For this review, use the dimensioned drawing (mm, ordinates from the lowest corner) and the shaded views. Coordinates: 2 decimals unless noted, no trailing zeros. Write each loop counter-clockwise with the first axis right and the second up, starting at its lowest first coordinate (ties: lowest second). Pieces come first, ordered by that corner, then holes. Notation, with made-up numbers: M 45,55.5 L 94,55.5 A33 cw 94,88.5 Z; hole C -25.5,-17.75 d10. An arc over 180 degrees is marked long. One line per question, with ' | ' between items.
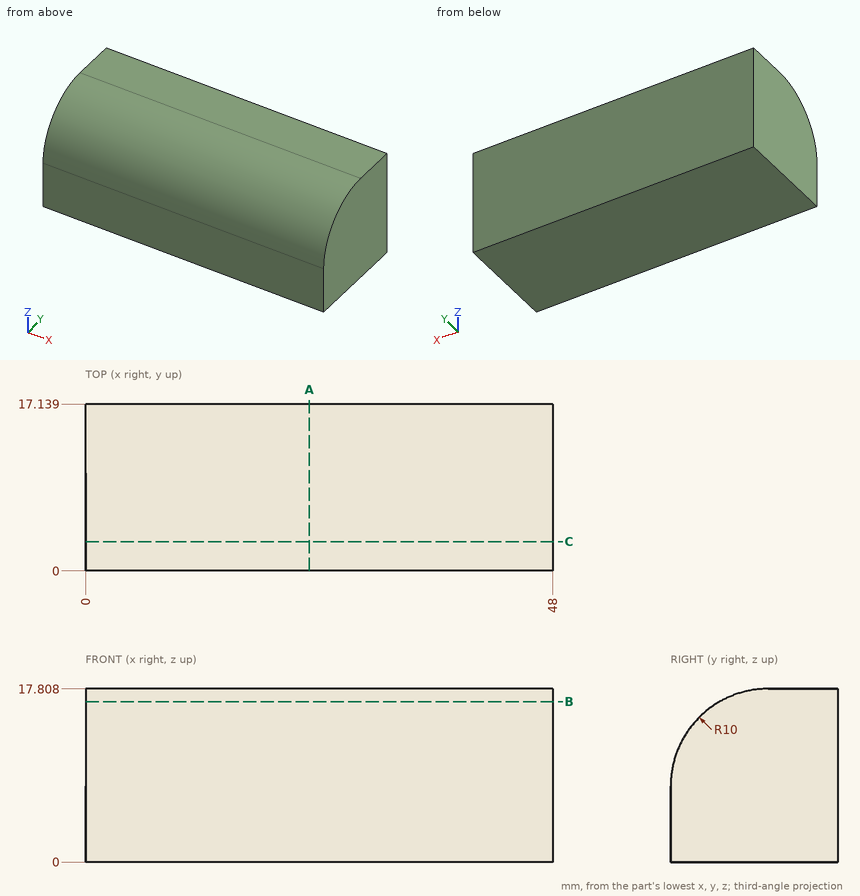
1. Take a section at C-C (y = 3). Write out the cut boundary in (x, z), then the cut area to 3 significant figures.
Answer sheet:
outline: M 0,0 L 48,0 L 48,14.95 L 0,14.95 Z | area: 718 mm^2
2. To check wall thickness, follow line 1 along Y through (x, z) = (25, 12); line 2 along Y through (x, z) = (4, 11); line 3 along Z through (x, y) = (28.5, 8.5) (1 decimal). State the ranges of each line that lie inside material, in increasing order. Write a range as [from, to].
Answer sheet:
line 1: [0.92, 17.14] | line 2: [0.52, 17.14] | line 3: [0, 17.7]
3. Take a section at B-B (z = 16.5). Write out the cut boundary in (x, y) (3 decimals), then the cut area to 3 significant figures.
Answer sheet:
outline: M 0,5.055 L 48,5.055 L 48,17.139 L 0,17.139 Z | area: 580 mm^2
4. Insertion check: pin 1 Ø3 at (x, y) = (20.5, 4.5) entering from +Z. The pin has a flat end and moves straight along its axis. Give the tip position at first contact, or say it passes through.
Answer sheet:
pin 1: z = 16.97
5. Take a section at A-A (x = 23). Write out the cut boundary in (y, z), then the cut area to 3 significant figures.
Answer sheet:
outline: M 0,0 L 17.14,0 L 17.14,17.81 L 10,17.81 A10 ccw 0,7.81 Z | area: 284 mm^2
